CAD build for the part. Positions are in the model's coordinates, mm. Coordinates: 2 decimals unless noted, no trailing zeros. Order: outer loops, then holes, each group sorted by start corner. A loop starts at its lowest first (then second) coordinate and runs counter-clockwise, first axis right, second up. Notation, with made-up numbers: M -14,-25.5 L -6,-25.5 A22 ccw -6,-4.5 Z; hole C -39,7.25 d8. An arc over 180 degrees is marked long. One line per item, written item: value.
from build123d import *

# Parameters (mm, degrees)
SKETCH_1_R          = 40
SKETCH_1_R_2        = 1.5
SKETCH_1_R_3        = 1.6
EXTRUDE_9_DEPTH     = 2
SKETCH_2_R          = 1.5
CUT_EXTRUDE_1_DEPTH = 2
FILLET_2_OUTLINE_R  = 1.5
FILLET_2_DEPTH      = 2


with BuildPart() as part:
    # 草图1 → 凸台-拉伸9 (new body)
    with BuildSketch(Plane(origin=(0, 0, 0), x_dir=(1, 0, 0), z_dir=(0, 1, 0))):
        with Locations(Location((0, 0, 0), (0, 0, 270))):
            Circle(SKETCH_1_R)
        with Locations(Location((-12.727922062, -5.656854248, 0), (0, 0, 270))):
            Circle(SKETCH_1_R_2, mode=Mode.SUBTRACT)
        with Locations(Location((-5.656854248, -12.727922062, 0), (0, 0, 270))):
            Circle(SKETCH_1_R_2, mode=Mode.SUBTRACT)
        with Locations(Location((-19.798989874, -12.727922061, 0), (0, 0, 270))):
            Circle(SKETCH_1_R_2, mode=Mode.SUBTRACT)
        with Locations(Location((-12.727922061, -19.798989874, 0), (0, 0, 270))):
            Circle(SKETCH_1_R_2, mode=Mode.SUBTRACT)
        with Locations(Location((4.949747468, 4.949747468, 0), (0, 0, 270))):
            Circle(SKETCH_1_R_2, mode=Mode.SUBTRACT)
        with Locations(Location((-4.949747468, 4.949747468, 0), (0, 0, 270))):
            Circle(SKETCH_1_R_2, mode=Mode.SUBTRACT)
        with Locations(Location((-4.949747468, -4.949747468, 0), (0, 0, 270))):
            Circle(SKETCH_1_R_2, mode=Mode.SUBTRACT)
        with Locations(Location((4.949747468, -4.949747468, 0), (0, 0, 270))):
            Circle(SKETCH_1_R_2, mode=Mode.SUBTRACT)
        with Locations(Location((35.582997469, 5.463541991, 0), (0, 0, 270))):
            Circle(SKETCH_1_R_3, mode=Mode.SUBTRACT)
        with Locations(Location((5.463541991, -35.582997469, 0), (0, 0, 270))):
            Circle(SKETCH_1_R_3, mode=Mode.SUBTRACT)
        with Locations(Location((-35.582997469, -5.463541991, 0), (0, 0, 270))):
            Circle(SKETCH_1_R_3, mode=Mode.SUBTRACT)
        with Locations(Location((-5.463541991, 35.582997469, 0), (0, 0, 270))):
            Circle(SKETCH_1_R_3, mode=Mode.SUBTRACT)
    extrude(amount=EXTRUDE_9_DEPTH)

    # 草图2 → 切除-拉伸1 (cut)
    with BuildSketch(Plane(origin=(0, 2, 0), x_dir=(1, 0, 0), z_dir=(0, 1, 0))):
        with Locations(Location((8.838834765, 15.909902577, 0), (0, 0, 270))):
            Circle(SKETCH_2_R)
        with Locations(Location((15.909902577, 8.838834765, 0), (0, 0, 270))):
            Circle(SKETCH_2_R)
        with Locations(Location((15.909902576, 22.980970389, 0), (0, 0, 270))):
            Circle(SKETCH_2_R)
        with Locations(Location((22.980970389, 15.909902576, 0), (0, 0, 270))):
            Circle(SKETCH_2_R)
    extrude(amount=-CUT_EXTRUDE_1_DEPTH, mode=Mode.SUBTRACT)

    # 圆角2: read off the stored shape, not the designer's step
    # 圆角2 outline → 圆角2 (add)
    with BuildSketch(Plane(origin=(0, 0, 0), x_dir=(1, 0, 0), z_dir=(0, 1, 0))):
        with BuildLine():
            ThreePointArc((-37.808106107, -13.059368767), (-37.573895805, -17.467074044), (-39.712873079, -21.32809677))
            Line((-39.712873079, -21.32809677), (-50.911688244, -32.526911935))
            ThreePointArc((-50.911688244, -32.526911935), (-53.254833995, -38.183766185), (-50.911688244, -43.840620434))
            Line((-50.911688244, -43.840620434), (-43.840620432, -50.911688246))
            ThreePointArc((-43.840620432, -50.911688246), (-38.183766183, -53.254833997), (-32.526911933, -50.911688246))
            Line((-32.526911933, -50.911688246), (-21.328096767, -39.71287308))
            ThreePointArc((-21.328096767, -39.71287308), (-17.467074041, -37.573895806), (-13.059368765, -37.808106108))
            ThreePointArc((-13.059368765, -37.808106108), (-28.284271247, -28.284271248), (-37.808106107, -13.059368767))
        make_face()
        with Locations((-38.18376618, -45.254833999)):
            Circle(FILLET_2_OUTLINE_R, mode=Mode.SUBTRACT)
        with Locations((-45.254833993, -38.183766188)):
            Circle(FILLET_2_OUTLINE_R, mode=Mode.SUBTRACT)
        with Locations((-31.112698372, -38.183766184)):
            Circle(FILLET_2_OUTLINE_R, mode=Mode.SUBTRACT)
        with Locations((-38.183766184, -31.112698372)):
            Circle(FILLET_2_OUTLINE_R, mode=Mode.SUBTRACT)
    extrude(amount=FILLET_2_DEPTH)


solid = part.part
Q1. Mould opens along X. For faces 1 (the face through (-37.002, 0.986, 6.202)), 2 (the face through (-38.272, 0.986, 53.254)), 3 (the face through (-53.254, 0.986, 38.096)) say: released by +X, released by -X, zero draft, split by the parting line, or undercut.
Recorded:
face 1: undercut
face 2: split by the parting line
face 3: released by -X
Q2. Slice it at A-A (y = 0.75). Give the number of separate pieces and of enclosed holes in the cut face, plus the area to 3 significant figures.
Recorded:
separate pieces: 1
enclosed holes: 20
area: 5,580 mm^2
Q3. Pin check, flat tips, straight feed: pin 1 Ø2.5 at (x, z) = (-45.25, 38.18) entering from +Y; pin 2 Ø1 at (x, y) = (4.5, 1.5) entering from +Z. Stop position of each tip, or through.
Recorded:
pin 1: passes through
pin 2: stops at z = 39.8
Q4. Drill centre lines: line 1 along Z through (x, y) = (15.5, 1.2); line 2 along X through (y, z) = (0.4, 19.5); line 3 along Z through (x, y) = (-46, 0.55). Where is each one in solid material? Low to high.
Recorded:
line 1: z = -36.87 to -24.42, -21.54 to -10.28, -7.4 to 36.87
line 2: x = -38.35 to -14.2, -11.26 to 34.92
line 3: z = 27.62 to 36.88, 39.49 to 48.75
Q5. Slice it at C-C (z = 0). List the corners of the cut face in (x, y).
Recorded:
outline: M -40,0 L 40,0 L 40,2 L -40,2 Z
Q6. Slice it at B-B (x = 0). List the corners of the cut face in (y, z), plus the area to 3 significant figures.
Recorded:
outline: M 0,-40 L 2,-40 L 2,40 L 0,40 Z
area: 160 mm^2
